Check sheet for the drawn part. Datum: minimum x, y, z corner. Units: mm. A direction names the side the tool comes from. Give positions to 0.01 mm unless a question says otherwise; leave off trailing zeros. Write each loop counter-clockwise with the first axis right and the second up, starting at its lowest first coordinate (ties: lowest second). Pieces come first, ordered by that corner, then holes. Notation, with made-up numbers: (86, -12) - (91, -12) arc R20 ccw to (91, 26) - close; hole circle Ø6 at (87.25, -26). An arc over 180 degrees is marked (long way). Return JSON: item names as keys, results as strings. Group by question number.
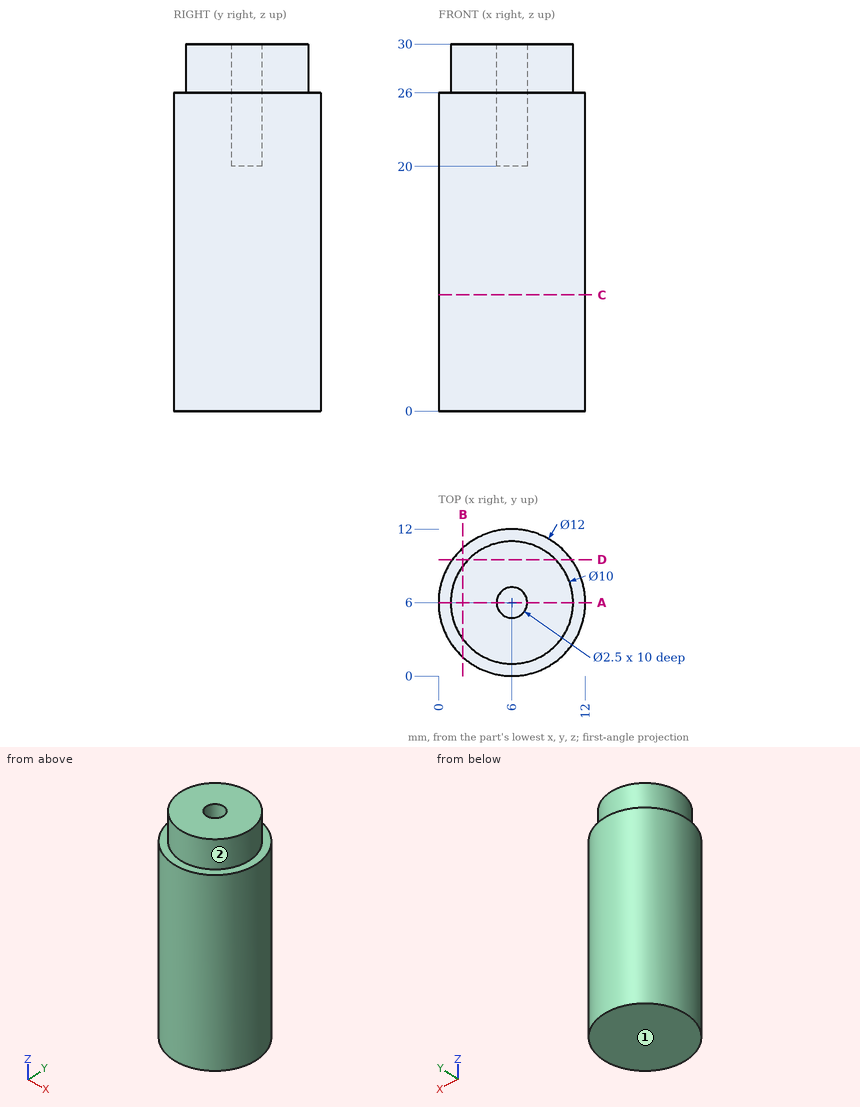
Item 1: Section check C-C on z = 9.5. Record the cut outline in (x, y).
Item 2: Depth check by flat-ended pin: pin 1 (2 mm diameter, centred on y = 8.5, z = 26.5, fed in from -X); pin 2 (1.2 mm diameter, centred on x = 6, y = 6, fed in from +Z). Enter the tip coordinate at first touch or a pass-through.
Item 3: Section check B-B on x = 2. Record the cut outline in (y, z).
Item 4: Access from +Z, -Z, +X, -X, +Y, -Y to the whole of each face (thin tool, end or side, straight path). Record for the marked faces 1 and 2.
Item 5: Material ranges on line 1 along Y through (x, z) = (6, 24.5); line 2 along Y through (x, z) = (6, 27); line 3 along Z through (x, y) = (0.5, 5), recorded low to high. Write a range as from..to.
Item 6: Section check D-D on y = 9.5. Record the cut outline in (x, z), plus the area to 3 significant figures.
Item 7: Section check A-A on y = 6. Record the cut outline in (x, z).
Reply:
{
 "1": {"outline": "circle Ø12 at (6, 6)"},
 "2": {"pin 1": "x = 0.23", "pin 2": "z = 20"},
 "3": {"outline": "(1.53, 0) - (10.47, 0) - (10.47, 26) - (9, 26) - (9, 30) - (3, 30) - (3, 26) - (1.53, 26) - close"},
 "4": {"face 1": "-Z, +X, -X, +Y, -Y", "face 2": "+Z"},
 "5": {"line 1": "0..4.75, 7.25..12", "line 2": "1..4.75, 7.25..11", "line 3": "0..26"},
 "6": {"outline": "(1.13, 0) - (10.87, 0) - (10.87, 26) - (9.57, 26) - (9.57, 30) - (2.43, 30) - (2.43, 26) - (1.13, 26) - close", "area": "282 mm²"},
 "7": {"outline": "(0, 0) - (12, 0) - (12, 26) - (11, 26) - (11, 30) - (7.25, 30) - (7.25, 20) - (4.75, 20) - (4.75, 30) - (1, 30) - (1, 26) - (0, 26) - close"}
}
